from build123d import *

# Parameters (mm, degrees)
F1_DEPTH      = 2.92
F2_W          = 11.3588606473
F2_H          = 3.0194446445
F3_DEPTH      = 4.064
F3_DEPTH_BACK = 1.778


with BuildPart() as f1:
    # F0 (on Front) → F1 (new body)
    with BuildSketch(Plane.XZ):
        Polygon((-21.565, 41.5), (-3.585, -41.5), (-3.585, 41.5), align=None)
        Polygon((-21.565, 41.5), (-3.585, 41.5), (3.5597670358, 41.5), (3.5597670358, 56.15), (-21.565, 56.15), align=None)
        Polygon((-21.565, 72.5), (-21.565, 56.15), (3.5597670358, 56.15), (-4.2378189974, 60.8550645411), (-14.3992334591, 65.134861098), (-14.3992334591, 71.3648572564), (-4.2378189974, 71.3648572564), (6.6109970212, 65.134861098), (16.8742514001, 65.134861098), (13.7305296957, 71.3648572564), (3.8987922017, 76.1159212991), (-14.3992334591, 76.1159212991), align=None)
        Polygon((-3.585, -41.5), (3.585, -41.5), (3.585, 41.5), (3.5597670358, 41.5), (-3.585, 41.5), align=None)
    extrude(amount=F1_DEPTH)

    # F2 (on Right) → F3 (join, two sides)
    with BuildSketch(Plane.YZ) as f3_sk:
        with Locations((-8.5862084525, -34.0649671853)):
            Rectangle(F2_W, F2_H)
    extrude(amount=-F3_DEPTH)
    extrude(f3_sk.sketch, amount=F3_DEPTH_BACK)


solid = f1.part
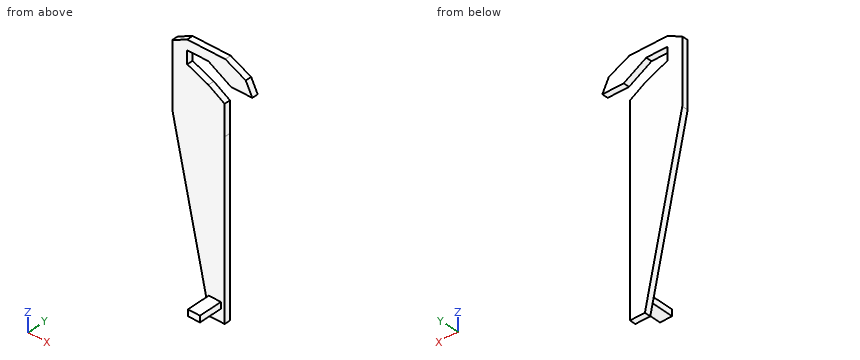
Read the model definition and answer for the solid it produces. Units are mm, in the model's axes. Round coordinates to 2 decimals unless told otherwise and drop trailing zeros. Write each loop counter-clockwise with the first axis right and the second up, starting at its lowest first coordinate (ties: lowest second). Pieces come first, ordered by that corner, then holes.
1. The part is cut by section D-D, the plane z = 17.5. Determine the outline of the cut face in (x, y) (3 decimals).
2. The part is cut by section A-A, the plane y = -1.25. Determine the outline of the cut face in (x, z) (3 decimals).
3. The part is cut by section C-C, the plane z = 68.5. Determine the outline of the cut face in (x, y) (3 decimals).
4. The part is cut by section B-B, the plane x = -6.5. Determine the outline of the cut face in (y, z).
5. Straight lines are drawn through the part: L1, parallel to Y at x = -8, z = 61; L2, parallel to Z at x = -1, y = -11; L3, parallel to X at y = -0.5, z = 67 (3 decimals). For each, find the intervals that lie inside material, in ascending order.
6. Given pin 1 Ø8 at (y, z) = (-3.5, 9.5) entering from -X; pin 2 Ø19 at (x, z) = (3.5, 35) entering from -Y; pin 3 Ø2.5 at (y, z) = (-2, 10) entering from +X (3 decimals); pin 4 Ø4 at (y, z) = (-6, -29) entering from +X, each flat-ended and moving along its own axis, determine where each tip first touches the part or whether it passes through.
Values:
1. outline: (-16.366, -2.92) - (3.585, -2.92) - (3.585, 0) - (-16.366, 0) - close
2. outline: (-21.565, 41.5) - (-3.585, -41.5) - (3.585, -41.5) - (3.585, 41.5) - (3.56, 41.5) - (3.56, 56.15) - (-4.238, 60.855) - (-14.399, 65.135) - (-14.399, 71.365) - (-4.238, 71.365) - (6.611, 65.135) - (16.874, 65.135) - (13.731, 71.365) - (3.899, 76.116) - (-14.399, 76.116) - (-21.565, 72.5) - close
3. outline: (-21.565, -2.92) - (-14.399, -2.92) - (-14.399, 0) - (-21.565, 0) - close; (0.751, -2.92) - (15.176, -2.92) - (15.176, 0) - (0.751, 0) - close
4. outline: (-2.92, -28.04) - (0, -28.04) - (0, 61.81) - (-2.92, 61.81) - close; (-2.92, 71.36) - (0, 71.36) - (0, 76.12) - (-2.92, 76.12) - close
5. L1: y = -2.92 to 0
5. L2: z = -35.57 to -32.56
5. L3: x = -21.565 to -14.399, 3.363 to 15.933
6. pin 1: stops at x = -15.49
6. pin 2: stops at y = -2.92
6. pin 3: stops at x = 3.585
6. pin 4: passes through
